Can you work these out from the model? Positions are in its coordinate system, mm. Face numbers are marked on the shaded views. A direction names the side the tool comes from. Round coordinates to 2 decimals unless told otherwise and drop trailing zeros. Loops run counter-clockwise (first coordinate to the right, second up) from the corner with the lowest first, then second, coordinate; pieces in that order, holes last.
(1) I want a section at C-C on x = -233. Write out the boundary of the cut face in (y, z), plus the area to 3 significant figures.
(2) Which directions (+Z, -Z, +X, -X, +Y, -Y) give clear straight access to the entire face, cutting with the end or side of a thin tool? Please do the marked faces 1, 2, 3 and 4.
(3) Will these pins go through, and if not, where does the flat tip stop? pin 1 Ø1.5 at (x, y) = (-5, 72) entering from +Z; pin 2 Ø4 at (y, z) = (-77, -462.5) entering from -X.
(4) I want a section at B-B on z = -657. Write out the boundary of the cut face in (x, y).
(5) Thinking about a two-plate mould opening in Z: for the marked faces 5, 6, 7 and 8, which applies, released by +Z, released by -Z, zero draft, split by the parting line, or undercut?
(6) If I drill on line 1 along X through (y, z) = (52, -479.5); line 2 along Z through (x, y) = (-141, 82); line 3 along Z through (x, y) = (130.5, 63.5), over which ranges is the centre line in solid material (lowest first)?
(7) I want a section at A-A on y = 88. Write out the boundary of the cut face in (x, z).
from build123d import *

# Parameters (mm, degrees)
BOSS_EXTRUDE1_DEPTH = 100


with BuildPart() as part:
    # Sketch1 → Boss-Extrude1 (new, symmetric)
    with BuildSketch(Plane(origin=(0, 0, 0), x_dir=(1, 0, 0), z_dir=(0, 1, 0))):
        with BuildLine():
            Line((-300, 0), (300, 0))
            Line((300, 0), (300, 192.264973081))
            ThreePointArc((300, 192.264973081), (286.602540378, 242.264973081), (250, 278.867513459))
            Line((250, 278.867513459), (170, 325.055534995))
            ThreePointArc((170, 325.055534995), (133.397459622, 361.658075373), (120, 411.658075373))
            Line((120, 411.658075373), (120, 512.501692217))
            ThreePointArc((120, 512.501692217), (127.612046749, 550.770035453), (149.289321881, 583.212370335))
            Line((149.289321881, 583.212370335), (170.710678119, 604.633726573))
            ThreePointArc((170.710678119, 604.633726573), (192.387953251, 637.076061455), (200, 675.344404691))
            Line((200, 675.344404691), (200, 800))
            Line((200, 800), (-200, 800))
            Line((-200, 800), (-200, 675.344404691))
            ThreePointArc((-200, 675.344404691), (-192.387953251, 637.076061455), (-170.710678119, 604.633726573))
            Line((-170.710678119, 604.633726573), (-149.289321881, 583.212370335))
            ThreePointArc((-149.289321881, 583.212370335), (-127.612046749, 550.770035453), (-120, 512.501692217))
            Line((-120, 512.501692217), (-120, 411.658075373))
            ThreePointArc((-120, 411.658075373), (-133.397459622, 361.658075373), (-170, 325.055534995))
            Line((-170, 325.055534995), (-250, 278.867513459))
            ThreePointArc((-250, 278.867513459), (-286.602540378, 242.264973081), (-300, 192.264973081))
            Line((-300, 192.264973081), (-300, 0))
        make_face()
    extrude(amount=BOSS_EXTRUDE1_DEPTH, both=True)


solid = part.part
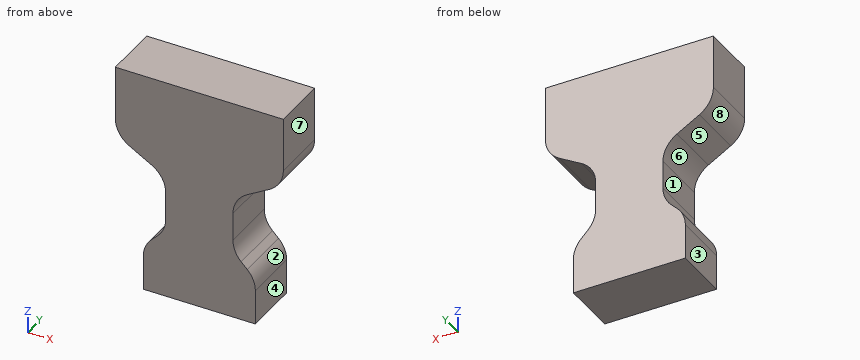
Filled sheet:
1. outline: (-100, -288.68) - (100, -288.68) - (100, 0) - (-100, 0) - close
1. area: 57,700 mm2
2. face 1: -X, +Y, -Y
2. face 2: +X, +Y, -Y
2. face 3: -Z, -X, +Y, -Y
2. face 4: -Z, +X, +Y, -Y
3. pin 1: stops at z = 0
3. pin 2: stops at x = -120
4. outline: (-198.3, -100) - (198.3, -100) - (198.3, 100) - (-198.3, 100) - close
5. face 5: undercut
5. face 6: undercut
5. face 7: zero draft
5. face 8: released by -Z
6. line 1: x = -120 to 120
6. line 2: z = -800 to -573.81, -350.35 to 0
6. line 3: z = -800 to -557.11, -367.05 to 0
7. outline: (-300, -192.26) arc R100 ccw to (-250, -278.87) - (-170, -325.06) arc R100 cw to (-120, -411.66) - (-120, -512.5) arc R100 cw to (-149.29, -583.21) - (-170.71, -604.63) arc R100 ccw to (-200, -675.34) - (-200, -800) - (200, -800) - (200, -675.34) arc R100 ccw to (170.71, -604.63) - (149.29, -583.21) arc R100 cw to (120, -512.5) - (120, -411.66) arc R100 cw to (170, -325.06) - (250, -278.87) arc R100 ccw to (300, -192.26) - (300, 0) - (-300, 0) - close
